```python
from build123d import *

# Parameters (mm, degrees)
F1_DEPTH      = 56.5685424949
F6_DEPTH      = 50
F6_DEPTH_BACK = 5
F7_DEPTH      = 25
F7_DEPTH_BACK = 50


with BuildPart() as f1:
    # F0 (on Top) → F1 (new body)
    with BuildSketch(Plane.XY):
        Polygon((20, -20), (20, 20), (-20, 20), align=None)
    extrude(amount=F1_DEPTH)

    # F4 (on face) → F6 (cut, two sides)
    with BuildSketch(Plane(origin=(10, -10, 14.1421356237), x_dir=(0.8660254038, 0.2886751346, -0.4082482905), z_dir=(-0.5, 0.5, -0.7071067812))) as f6_sk:
        Polygon((-20.8771324027, -29.5247237874), (-28.3771324027, -40.1313255052), (-18.3771324027, -36.5957915992), align=None)
        Polygon((2.7831216351, 3.9359283621), (-4.7168783649, -6.6706733557), (5.2831216351, -3.1351394497), align=None)
    extrude(amount=F6_DEPTH, mode=Mode.SUBTRACT)
    extrude(f6_sk.sketch, amount=-F6_DEPTH_BACK, mode=Mode.SUBTRACT)

    # F4 (on face) → F7 (cut, two sides)
    with BuildSketch(Plane(origin=(10, -10, 14.1421356237), x_dir=(0.8660254038, 0.2886751346, -0.4082482905), z_dir=(-0.5, 0.5, -0.7071067812))) as f7_sk:
        Polygon((-11.5470053838, -16.3299316186), (-16.5470053838, -23.4009994304), (-6.5470053838, -19.8654655245), (-9.0470053838, -12.7943977126), align=None)
    extrude(amount=-F7_DEPTH, mode=Mode.SUBTRACT)
    extrude(f7_sk.sketch, amount=F7_DEPTH_BACK, mode=Mode.SUBTRACT)


solid = f1.part
```
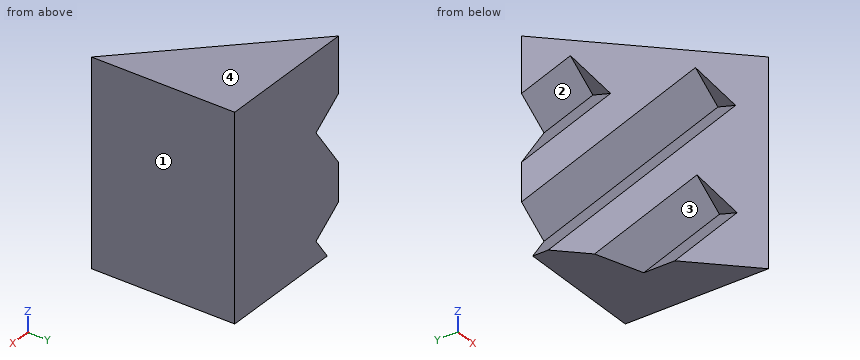
Geometry check sheet. Reference: the model listing, model coordinates, mm. Face numbers are marked on the shaded views. Coordinates: 2 decimals unless noted, no trailing zeros. Loops run counter-clockwise (first coordinate to the right, second up) from the corner with the lowest first, then second, coordinate; pieces in that order, holes last. Notation, with made-up numbers: (85, -10.5) - (135, -10.5) arc R18 cw to (135, 0.5) - close; hole circle Ø6 at (-4, -10). An arc over 180 degrees is marked (long way). One line per item, written item: value. Start each with the question number.
(1) Mould release check, pull along Z, two halves, no side actions. Record for the marked faces 1, 2, 3 and 4: released by +Z, released by -Z, zero draft, split by the parting line, or undercut.
(2) Depth check by flat-ended pin: P1, Ø10, axis at x = 10.5, z = 22, coming from the -Y side; P2, Ø8, axis at x = 4, y = -11.5, coming from the -Z side; P3, Ø8, axis at x = -4.5, z = 28, coming from the -Y side; P4, Ø10, axis at y = -8.5, z = 34, coming from the -X side. Enter the tip coordinate at first touch or a pass-through.
(3) Cross-section at C-C on y = 0. Enter the section's corners in (x, z), plus the area to 3 significant figures.
(4) Cross-section at D-D on x = 1.5. Enter the section's corners in (y, z).
(5) Cross-section at A-A on x = -14. Enter the section's corners in (y, z), plus the area to 3 significant figures.
(6) Cross-section at B-B on z = 30. Enter the section's corners in (x, y).
(7) Material ranges on line 1 (Z direction, x = -6.5, y = 7); line 2 (Z direction, x = -2.5, y = 4); line 3 (Z direction, x = -8.5, y = 13), recorded low to high. Write a range as [from, to].
Results below:
1. face 1: zero draft
1. face 2: undercut
1. face 3: undercut
1. face 4: released by +Z
2. P1: stops at y = -15.5
2. P2: passes through
2. P3: stops at y = 5.1
2. P4: stops at x = 5.53
3. outline: (0, 11.55) - (8.66, 5.43) - (4.82, 0) - (20, 0) - (20, 56.57) - (0, 56.57) - (0, 40.53) - (8.66, 34.41) - (0, 22.16) - close
3. area: 989 mm2
4. outline: (-1.5, 13.68) - (4.95, 0) - (20, 0) - (20, 56.57) - (-1.5, 56.57) - (-1.5, 42.65) - (7.16, 24.28) - (-1.5, 24.28) - close
5. outline: (14, 0) - (20, 0) - (20, 2.36) - (14, 2.36) - close; (14, 20.73) - (20, 8) - (20, 31.34) - (14, 31.34) - close; (14, 49.71) - (20, 36.98) - (20, 56.57) - (14, 56.57) - close
5. area: 195 mm2
6. outline: (-14.95, 14.95) - (-7.45, 7.45) - (5.54, 3.12) - (5.54, -5.54) - (20, -20) - (20, 20) - (-14.95, 20) - close
7. line 1: z = [1.3, 12.97], [30.28, 41.95], [44.9, 56.57]
7. line 2: z = [4.84, 18.63], [33.81, 56.57]
7. line 3: z = [0, 10.14], [18.96, 39.12], [47.94, 56.57]
